```python
from build123d import *

# Parameters (mm, degrees)
BOSS_EXTRUDE1_START = 6
SKETCH2_R           = 72.5
SKETCH2_R_2         = 3
BOSS_EXTRUDE1_DEPTH = 3


with BuildPart() as part:
    # Sketch1 → Revolve1 (revolve)
    with BuildSketch(Plane(origin=(0, 0, 0), x_dir=(0, 0, -1), z_dir=(1, 0, 0)), mode=Mode.PRIVATE) as revolve1_sk:
        Polygon((0, 0), (0, -40), (22.5, -40), (22.5, 0), (50, 0), (50, 6), (0, 6), align=None)
    revolve(revolve1_sk.sketch.rotate(Axis((0, 6, 0), (0, -1, 0)), 180), axis=Axis((0, 6, 0), (0, -1, 0)))

    # Sketch2 → Boss-Extrude1 (add)
    with BuildSketch(Plane(origin=(0, 0, 0), x_dir=(1, 0, 0), z_dir=(0, 1, 0)).offset(BOSS_EXTRUDE1_START)):
        with Locations(Location((0, 0, 0), (0, 0, 90))):
            Circle(SKETCH2_R)
        with Locations(Location((0, -65, 0), (0, 0, 90))):
            Circle(SKETCH2_R_2, mode=Mode.SUBTRACT)
        with Locations(Location((-32.5, -56.291651246, 0), (0, 0, 90))):
            Circle(SKETCH2_R_2, mode=Mode.SUBTRACT)
        with Locations(Location((-56.291651246, -32.5, 0), (0, 0, 90))):
            Circle(SKETCH2_R_2, mode=Mode.SUBTRACT)
        with Locations(Location((-65, 0, 0), (0, 0, 90))):
            Circle(SKETCH2_R_2, mode=Mode.SUBTRACT)
        with Locations(Location((-56.291651246, 32.5, 0), (0, 0, 90))):
            Circle(SKETCH2_R_2, mode=Mode.SUBTRACT)
        with Locations(Location((-32.5, 56.291651246, 0), (0, 0, 90))):
            Circle(SKETCH2_R_2, mode=Mode.SUBTRACT)
        with Locations(Location((0, 65, 0), (0, 0, 90))):
            Circle(SKETCH2_R_2, mode=Mode.SUBTRACT)
        with Locations(Location((32.5, 56.291651246, 0), (0, 0, 90))):
            Circle(SKETCH2_R_2, mode=Mode.SUBTRACT)
        with Locations(Location((56.291651246, 32.5, 0), (0, 0, 90))):
            Circle(SKETCH2_R_2, mode=Mode.SUBTRACT)
        with Locations(Location((65, 0, 0), (0, 0, 90))):
            Circle(SKETCH2_R_2, mode=Mode.SUBTRACT)
        with Locations(Location((56.291651246, -32.5, 0), (0, 0, 90))):
            Circle(SKETCH2_R_2, mode=Mode.SUBTRACT)
        with Locations(Location((32.5, -56.291651246, 0), (0, 0, 90))):
            Circle(SKETCH2_R_2, mode=Mode.SUBTRACT)
    extrude(amount=-BOSS_EXTRUDE1_DEPTH)


solid = part.part
```
Geometry check sheet. Reference: the model listing, model coordinates, mm. A direction names the side the tool comes from. Round coordinates to 2 decimals unless told otherwise and drop trailing zeros. Order: outer loops, then holes, each group sorted by start corner. A loop starts at its lowest first (then second) coordinate and runs counter-clockwise, first axis right, second up. Notation, with made-up numbers: M -32.5,-4.5 L -4.5,-4.5 A14 ccw -4.5,7.5 Z; hole C 5.25,-25.75 d3. An arc over 180 degrees is marked long. Answer as CSV lines item,"result".
1) Sectioned sample at D-D on x = -39. Record the cut outline in (y, z).
Entries:
outline,"M 0,-31.29 L 3,-31.29 L 3,-61.12 L 6,-61.12 L 6,61.12 L 3,61.12 L 3,31.29 L 0,31.29 Z"
2) Sectioned sample at C-C on y = -21.5. Record the cut outline in (x, z).
Entries:
outline,"C 0,0 d45"
3) Gauge pin test, flat ends, axial feed: pin 1 Ø7 at (x, z) = (0, -65) entering from -Y; pin 2 Ø1 at (y, z) = (-4, -19) entering from -X; pin 3 Ø5 at (x, z) = (-33.5, 15.5) entering from -Y; pin 4 Ø7 at (x, z) = (-56.29, 32.5) entering from +Y. Record the tip position at first contact, or that the pin passes through.
Entries:
pin 1,"y = 3"
pin 2,"x = -12.81"
pin 3,"y = 0"
pin 4,"y = 6"
4) Tool access check on faces 4 (the face through (19.961, -19.72, 10.382)), 5 (the face through (0, -40, 0)). Record the directions out of +Z, -Z, +X, -X, +Y, -Y that give a thin tool (end or side, any length) a straight path to the whole face; none if there is none.
Entries:
face 4,"-Y"
face 5,"+Z, -Z, +X, -X, -Y"
5) Sectioned sample at B-B on z = -65. Record the cut outline in (x, y).
Entries:
outline,"M -32.11,3 L -3,3 L -3,6 L -32.11,6 Z; M 3,3 L 32.11,3 L 32.11,6 L 3,6 Z"
6) Thickness scan on probe 1 along X at (y, z) = (3.7, 0); probe 2 along Z at (x, y) = (57.5, 4); probe 3 along Y at (x, z) = (4, 27). Record the ranges inside material, lowest first. Write a range as [from, to].
Entries:
probe 1,"[-72.5, -68], [-62, 62], [68, 72.5]"
probe 2,"[-44.16, -35.25], [-29.75, 29.75], [35.25, 44.16]"
probe 3,"[0, 6]"
7) Mould release check, pull along X, two halves, no side actions. Record for faces 1 (the face through (-53.363, 4.521, 33.15)), 2 (the face through (-15.02, 1.52, 47.69)), 3 (the face through (47.3, 3, 17.1)): +X half, -X half, draft (parallel to the pull), parting line (faces both ways), or undercut.
Entries:
face 1,"undercut"
face 2,"parting line"
face 3,"draft"
8) Sectioned sample at A-A on x = -65. Record the cut outline in (y, z), and give its area (3 significant figures).
Entries:
outline,"M 3,-32.11 L 6,-32.11 L 6,-3 L 3,-3 Z; M 3,3 L 6,3 L 6,32.11 L 3,32.11 Z"
area,"175 mm2"
